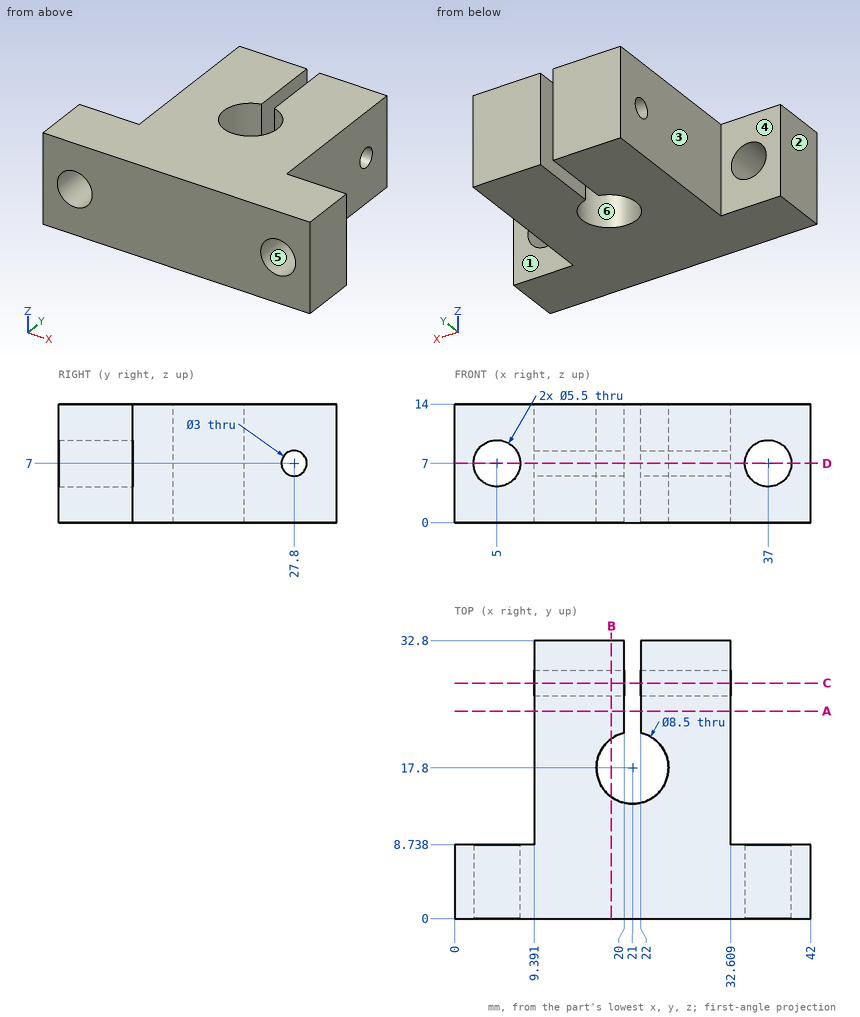
Job drawing, mm, ordinate dimensions from the low corner. One solid piece. A direction names the side the tool comes from. Give positions to 0.01 mm unless a question says otherwise; leave off trailing zeros. Loops run counter-clockwise (first coordinate to the right, second up) from the corner with the lowest first, then second, coordinate; pieces in that order, holes last. Notation, with made-up numbers: M 38.5,1.25 L 97.5,1.25 A20 cw 97.5,5.25 Z; hole C 27.5,-30.75 d3. An arc over 180 degrees is marked long. Answer in a Markdown table with one row per item. Add a question column.
Item 1: Band-saw the part on B-B on x = 18.5. Give the cut face in (y, z), then the cut area to 3 significant figures.
Item 2: Probe probe 1 along Y at (x, z) = (28, 7); probe 2 along X at (y, z) = (30, 5.5); probe 3 along X at (y, z) = (5, 5.25). List the from-to ranges inside material, lowest first.
Item 3: Drop flat-ended pins along their axis: P1, Ø5.5, axis at y = 25.5, z = 10.5, coming from the +X side; P2, Ø1.8, axis at y = 27.8, z = 7, coming from the -X side; P3, Ø6.5, axis at x = 5, z = 7, coming from the +Y side. Give the stop position or say it passes through.
Item 4: Band-saw the part on A-A on y = 24.5. Give the cut face in (x, z), then the cut area to 3 significant figures.
Item 5: Tool access for the marked faces 1, 2 and 3: list every direction of +Z, -Z, +X, -X, +Y, -Y with a clear straight run to the whole face (end or side of a thin tool).
Item 6: Band-saw the part on D-D on z = 7. Give the cut face in (x, y).
Item 7: Mould opens along Y. For the marked faces 4, 5 and 6 say: +Y half, -Y half, draft (parallel to the pull), parting line (faces both ways), or undercut.
Item 8: Band-saw the part on C-C on y = 27.8. Give the cut face in (x, z).
Reply:
| question | item | result |
|---|---|---|
| 1 | outline | M 0,0 L 14.36,0 L 14.36,14 L 0,14 Z; M 21.24,0 L 32.8,0 L 32.8,14 L 21.24,14 Z; hole C 27.8,7 d3 |
| 1 | area | 356 mm^2 |
| 2 | probe 1 | y = 0 to 26.3, 29.3 to 32.8 |
| 2 | probe 2 | x = 9.39 to 20, 22 to 32.61 |
| 2 | probe 3 | x = 0 to 2.88, 7.12 to 34.88, 39.12 to 42 |
| 3 | P1 | stops at x = 32.61 |
| 3 | P2 | passes through |
| 3 | P3 | stops at y = 8.74 |
| 4 | outline | M 9.39,0 L 20,0 L 20,14 L 9.39,14 Z; M 22,0 L 32.61,0 L 32.61,14 L 22,14 Z |
| 4 | area | 297 mm^2 |
| 5 | face 1 | +Z, -Z, +X, +Y |
| 5 | face 2 | +Z, -Z, -X, +Y, -Y |
| 5 | face 3 | +Z, -Z, -X, +Y |
| 6 | outline | M 0,0 L 2.25,0 L 2.25,8.74 L 0,8.74 Z; M 7.75,0 L 34.25,0 L 34.25,8.74 L 32.61,8.74 L 32.61,26.3 L 22,26.3 L 22,21.93 A4.25 cw long 20,21.93 L 20,26.3 L 9.39,26.3 L 9.39,8.74 L 7.75,8.74 Z; M 9.39,29.3 L 20,29.3 L 20,32.8 L 9.39,32.8 Z; M 22,29.3 L 32.61,29.3 L 32.61,32.8 L 22,32.8 Z; M 39.75,0 L 42,0 L 42,8.74 L 39.75,8.74 Z |
| 7 | face 4 | +Y half |
| 7 | face 5 | draft |
| 7 | face 6 | undercut |
| 8 | outline | M 9.39,0 L 20,0 L 20,5.5 L 9.39,5.5 Z; M 9.39,8.5 L 20,8.5 L 20,14 L 9.39,14 Z; M 22,0 L 32.61,0 L 32.61,5.5 L 22,5.5 Z; M 22,8.5 L 32.61,8.5 L 32.61,14 L 22,14 Z |
